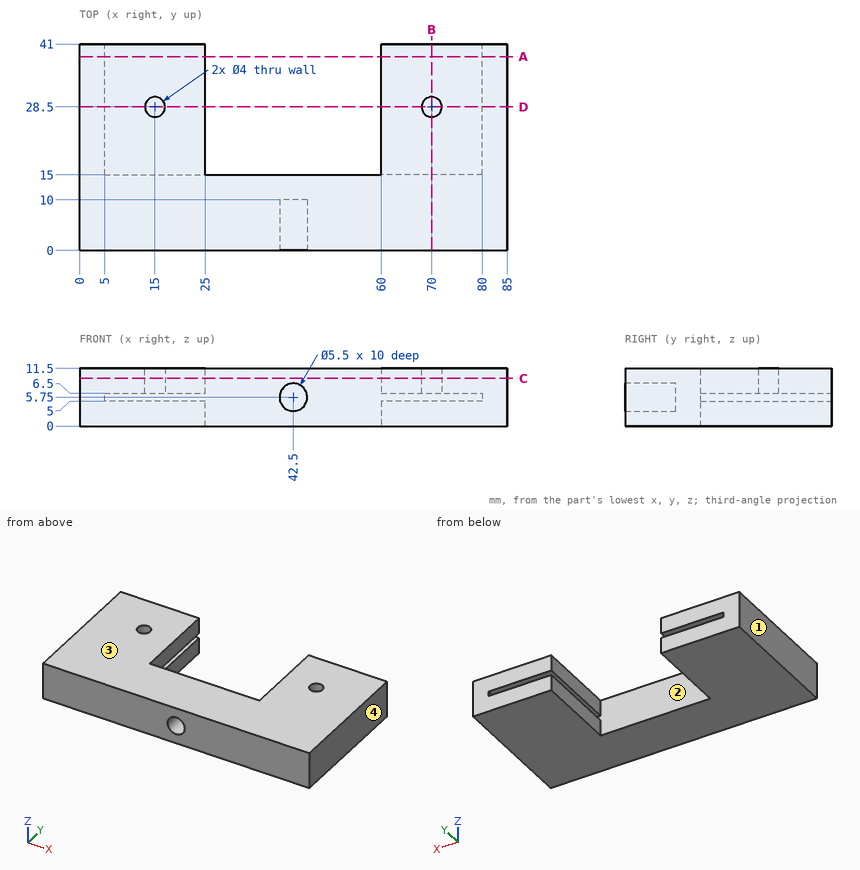
Input: dimensioned drawing with shaded views. Units: mm. Origin: part minimum x, y, z. Give positions to 0.01 mm unless a question says otherwise; leave off trailing zeros. Write each loop counter-clockwise with the first axis right and the second up, starting at its lowest first coordinate (ties: lowest second). Pieces come first, ordered by that corner, then holes. Notation, with made-up numbers: M 45,54 L 95,54 A22 ccw 95,86 Z; hole C 80.25,74.5 d5. An arc over 180 degrees is marked long. Write item = value, one per line. Start each with the question number.
1) Draft query along X for the marked faces 1, 2, 3 and 4. Return one class per face: +X half, -X half, draft (parallel to the pull), parting line (faces both ways), or undercut.
2) Cut plane B-B on x = 70. Return the cut outline in (y, z).
3) First-contact query: pin 1 Ø3.5 at (x, z) = (42.5, 5.75) entering from -Y; pin 2 Ø5 at (x, z) = (28.5, 4) entering from +Y. Flat tips, straight axial feed; report the tip coordinate or a pass-through.
4) Material intervals for line 1 along Y through (x, z) = (70, 9.15); line 2 along X through (y, z) = (19.5, 7); line 3 along X through (y, z) = (4, 5.75), sorted ascending. Write a range as [from, to].
5) Cut plane D-D on y = 28.5. Return the cut outline in (x, z), then the cut area to 3 significant figures.
6) Cut plane C-C on z = 9.5. Return the cut outline in (x, y), then the cut area to 3 significant figures.
7) Cut plane A-A on y = 38.5. Return the cut outline in (x, z), then the cut area to 3 significant figures.
Solved:
q1.face_1 = -X half
q1.face_2 = undercut
q1.face_3 = draft
q1.face_4 = +X half
q2.outline = M 0,0 L 41,0 L 41,5 L 15,5 L 15,6.5 L 26.5,6.5 L 26.5,11.5 L 0,11.5 Z; M 30.5,6.5 L 41,6.5 L 41,11.5 L 30.5,11.5 Z
q3.pin_1 = 10
q3.pin_2 = 15
q4.line_1 = [0, 26.5], [30.5, 41]
q4.line_2 = [0, 25], [60, 85]
q4.line_3 = [0, 39.75], [45.25, 85]
q5.outline = M 0,0 L 25,0 L 25,5 L 5,5 L 5,6.5 L 13,6.5 L 13,11.5 L 0,11.5 Z; M 17,6.5 L 25,6.5 L 25,11.5 L 17,11.5 Z; M 60,0 L 85,0 L 85,11.5 L 72,11.5 L 72,6.5 L 80,6.5 L 80,5 L 60,5 Z; M 60,6.5 L 68,6.5 L 68,11.5 L 60,11.5 Z
q5.area = 475 mm2
q6.outline = M 0,0 L 85,0 L 85,41 L 60,41 L 60,15 L 25,15 L 25,41 L 0,41 Z; hole C 15,28.5 d4; hole C 70,28.5 d4
q6.area = 2,550 mm2
q7.outline = M 0,0 L 25,0 L 25,5 L 5,5 L 5,6.5 L 25,6.5 L 25,11.5 L 0,11.5 Z; M 60,0 L 85,0 L 85,11.5 L 60,11.5 L 60,6.5 L 80,6.5 L 80,5 L 60,5 Z
q7.area = 515 mm2
